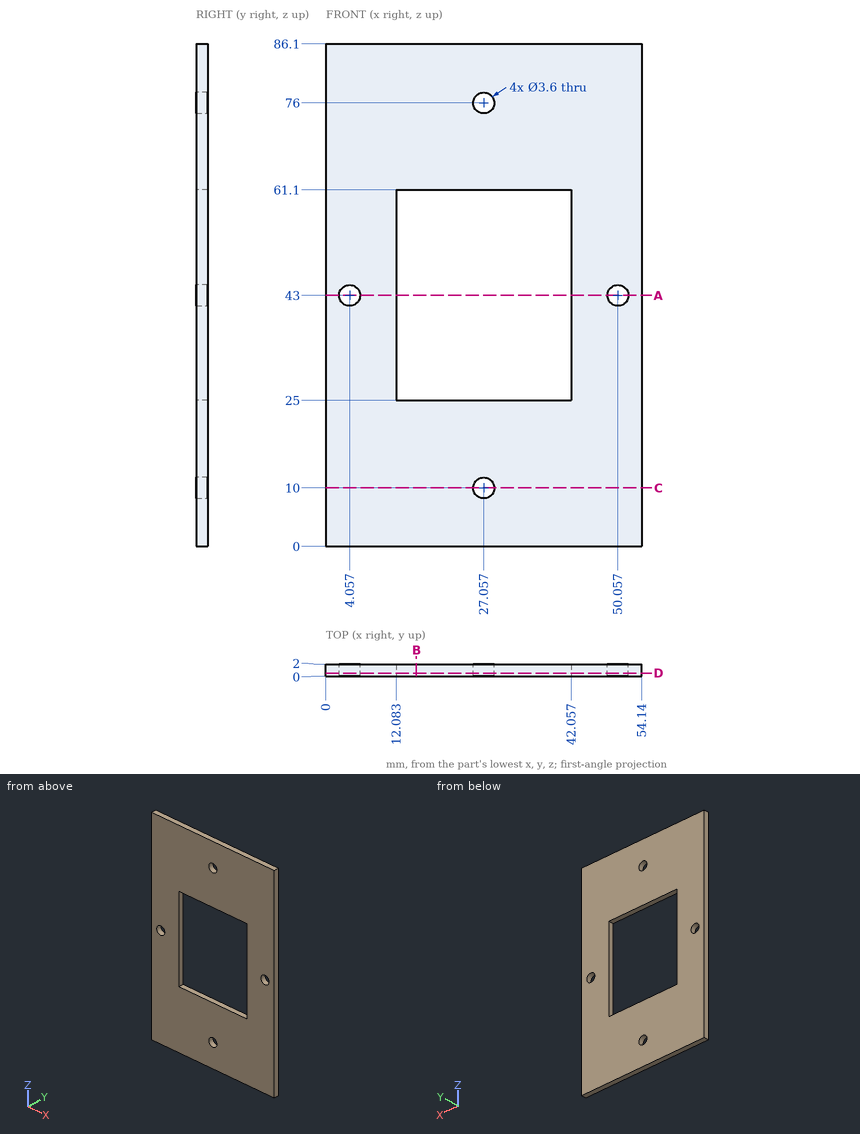
Can you work these out from the drawing? Everything is in mm from the part's minimum corner. Coordinates: 2 decimals unless noted, no trailing zeros. Write each loop counter-clockwise with the first axis right and the second up, starting at its lowest first coordinate (ties: lowest second). Pieces come first, ordered by that corner, then holes. Notation, with made-up numbers: (-27.5, 69.25) - (-2.5, 69.25) arc R21 cw to (-2.5, 80.25) - close; hole circle Ø5 at (2.5, -19). An arc over 180 degrees is marked (long way). One line per item, written item: value.
1) I need wall thicknesses on line 1 along X through (y, z) = (1.25, 43); line 2 along X through (y, z) = (0.65, 31.5); line 3 along Z through (x, y) = (16, 0.2). Which ranges of each line are inside material? Lowest first, please.
Model answer:
line 1: x = 0 to 2.26, 5.86 to 12.08, 42.06 to 48.26, 51.86 to 54.14
line 2: x = 0 to 12.08, 42.06 to 54.14
line 3: z = 0 to 25, 61.1 to 86.1
2) I'm going to push flat-ended pins straight in: P1, Ø3, axis at x = 50.06, z = 43, coming from the +Y side; P2, Ø4.5, axis at x = 27.06, z = 76, coming from the +Y side. Where does each tip first touch, or does it pass through?
Model answer:
P1: passes through
P2: stops at y = 2
3) Suppose I cut it at B-B on x = 15.5. Write out the boundary of the cut face in (y, z), and give its area (3 significant figures).
Model answer:
outline: (0, 0) - (2, 0) - (2, 25) - (0, 25) - close; (0, 61.1) - (2, 61.1) - (2, 86.1) - (0, 86.1) - close
area: 100 mm²
4) Suppose I cut it at D-D on y = 0.5. Write out the boundary of the cut face in (x, z), and give its area (3 significant figures).
Model answer:
outline: (0, 0) - (54.14, 0) - (54.14, 86.1) - (0, 86.1) - close; hole circle Ø3.6 at (4.06, 43); hole (12.08, 25) - (42.06, 25) - (42.06, 61.1) - (12.08, 61.1) - close; hole circle Ø3.6 at (27.06, 10); hole circle Ø3.6 at (27.06, 76); hole circle Ø3.6 at (50.06, 43)
area: 3,540 mm²
5) Suppose I cut it at A-A on z = 43. Write out the boundary of the cut face in (x, y).
Model answer:
outline: (0, 0) - (2.26, 0) - (2.26, 2) - (0, 2) - close; (5.86, 0) - (12.08, 0) - (12.08, 2) - (5.86, 2) - close; (42.06, 0) - (48.26, 0) - (48.26, 2) - (42.06, 2) - close; (51.86, 0) - (54.14, 0) - (54.14, 2) - (51.86, 2) - close
6) Suppose I cut it at C-C on z = 10. Write out the boundary of the cut face in (x, y), and give its area (3 significant figures).
Model answer:
outline: (0, 0) - (25.26, 0) - (25.26, 2) - (0, 2) - close; (28.86, 0) - (54.14, 0) - (54.14, 2) - (28.86, 2) - close
area: 101 mm²
